Here's how the part is built. I have some questions about the finished solid (model axes, mm). Round coordinates to 2 decimals unless told otherwise and drop trailing zeros. Loops run counter-clockwise (first coordinate to the right, second up) from the corner with the lowest first, then second, coordinate; pieces in that order, holes last. Notation, with made-up numbers: M -34,-20.5 L 13,-20.5 A33 cw 13,14.5 Z; hole C 13.5,-16 d2. An arc over 180 degrees is marked long. Answer as a JSON object with one key per item and string values.
from build123d import *

# Parameters (mm, degrees)
SKIZZE1_W                       = 20
SKIZZE1_H                       = 20
AUFSATZ_LINEAR_AUSTRAGEN1_DEPTH = 300
SCHNITT_LINEAR_AUSTRAGEN1_DEPTH = 302.330383466


with BuildPart() as part:
    # Skizze1 → Aufsatz-Linear austragen1 (new body)
    with BuildSketch(Plane(origin=(0, 0, 0), x_dir=(1, 0, 0), z_dir=(0, 1, 0))):
        with Locations((10, 10)):
            Rectangle(SKIZZE1_W, SKIZZE1_H)
    extrude(amount=AUFSATZ_LINEAR_AUSTRAGEN1_DEPTH)

    # Skizze2 → Schnitt-Linear austragen1 (cut, through all)
    with BuildSketch(Plane(origin=(0, 300, 0), x_dir=(1, 0, 0), z_dir=(0, 1, 0))):
        Polygon((7, 20), (10, 17), (13, 20), align=None)
        Polygon((20, 13), (17, 10), (20, 7), align=None)
        Polygon((0, 7), (0, 13), (3, 10), align=None)
        Polygon((7, 0), (13, 0), (10, 3), align=None)
    extrude(amount=-SCHNITT_LINEAR_AUSTRAGEN1_DEPTH, mode=Mode.SUBTRACT)


solid = part.part
Item 1: I want a section at A-A, the plane y = 93. Please give me the cut outline in (x, z), then the cut area to 3 significant figures.
Resolved:
{"outline": "M 0,-20 L 7,-20 L 10,-17 L 13,-20 L 20,-20 L 20,-13 L 17,-10 L 20,-7 L 20,0 L 13,0 L 10,-3 L 7,0 L 0,0 L 0,-7 L 3,-10 L 0,-13 Z", "area": "364 mm²"}
Item 2: Please list where these lines run through material, in increasing order: probe 1 along X at (y, z) = (42, -2); probe 2 along X at (y, z) = (224.5, -18.5); probe 3 along Z at (x, y) = (2.25, 29.5). Write a range as from..to.
Resolved:
{"probe 1": "0..9, 11..20", "probe 2": "0..8.5, 11.5..20", "probe 3": "-20..-10.75, -9.25..0"}
Item 3: I'm going to push a flat-ended pin straight in: pin 1 Ø4 at (y, z) = (190.5, -10) entering from -X. Where does the tip first touch, or does it pass through?
Resolved:
{"pin 1": "x = 1"}
